```python
from build123d import *

# Parameters (mm, degrees)
CIRCLE014_R      = 1.4
EXTRUDE175_DEPTH = 2
CIRCLE_R         = 2.9
EXTRUDE174_DEPTH = 2


with BuildPart() as extrude175:
    # Circle014 → Extrude175 (new body)
    with BuildSketch(Plane(origin=(-18.702098, -10.934014, -1), x_dir=(1, 0, 0), z_dir=(0, 0, 1))):
        Circle(CIRCLE014_R)
    extrude(amount=-EXTRUDE175_DEPTH)


with BuildPart() as cut087:
    # Circle → Extrude174 (new body)
    with BuildSketch(Plane(origin=(-18.702098, -10.934014, -3), x_dir=(1, 0, 0), z_dir=(0, 0, 1))):
        Circle(CIRCLE_R)
    extrude(amount=EXTRUDE174_DEPTH)

    # Cut087: cut Extrude175
    add(extrude175.part, mode=Mode.SUBTRACT)


solid = cut087.part
```
Geometry: final body of the model. Coordinates: model frame, mm. Coordinates: 2 decimals unless noted, no trailing zeros. Order: outer loops, then holes, each group sorted by start corner. A loop starts at its lowest first (then second) coordinate and runs counter-clockwise, first axis right, second up. Notation, with made-up numbers: (4.25, 41) - (29.25, 41) arc R25 ccw to (29.25, 55) - close; hole circle Ø8 at (48, -13.5). An arc over 180 degrees is marked (long way). Return JSON: item names as keys, results as strings. Group by question number.
1. Cut plane C-C (z = -1.2). Output: boundary loops of the cut face in (x, y).
2. Material intervals for line 1 along Y through (x, z) = (-19.65, -2.4); line 2 along Y through (x, z) = (-18.2, -1.55); line 3 along X through (y, z) = (-9.7, -1.95), sorted ascending. Write a range as [from, to].
3. Pull-direction query (Y, two-part tool) for faces 1 (the face through (-18.1, -12.2, -2)), 2 (the face through (-19.331, -13.765, -2.014)), 3 (the face through (-17, -10, -3)); classes: pulls with the +Y half, pulls with the -Y half, needs draft (parallel to the pull), parting line crosses it, or undercut.
4. Cut plane D-D (y = -9.3). Output: boundary loops of the cut face in (x, z).
5. Pin query (flat end, axial travel): pin 1 (1 mm diameter, centred on x = -21, z = -2, fed in from +Y); pin 2 (2.5 mm diameter, centred on x = -18.7, y = -10.93, fed in from -Z). Return the tip coordinate at first contact, or that it passes through.
6. Cut plane B-B (y = -10.2). Output: boundary loops of the cut face in (x, z), plus the area to 3 significant figures.
7. Cut plane A-A (x = -17.5). Output: boundary loops of the cut face in (y, z), plus the area to 3 significant figures.
Resolved:
{
 "1": {"outline": "circle Ø5.8 at (-18.7, -10.93); hole circle Ø2.8 at (-18.7, -10.93)"},
 "2": {"line 1": "y = [-13.67, -11.96], [-9.9, -8.19]", "line 2": "y = [-13.79, -12.24], [-9.63, -8.08]", "line 3": "x = [-21.33, -19.36], [-18.04, -16.08]"},
 "3": {"face 1": "undercut", "face 2": "parting line crosses it", "face 3": "needs draft"},
 "4": {"outline": "(-21.1, -3) - (-16.31, -3) - (-16.31, -1) - (-21.1, -1) - close"},
 "5": {"pin 1": "stops at y = -8.66", "pin 2": "passes through"},
 "6": {"outline": "(-21.51, -3) - (-19.89, -3) - (-19.89, -1) - (-21.51, -1) - close; (-17.51, -3) - (-15.9, -3) - (-15.9, -1) - (-17.51, -1) - close", "area": "6.45 mm²"},
 "7": {"outline": "(-13.57, -3) - (-11.65, -3) - (-11.65, -1) - (-13.57, -1) - close; (-10.22, -3) - (-8.29, -3) - (-8.29, -1) - (-10.22, -1) - close", "area": "7.69 mm²"}
}
